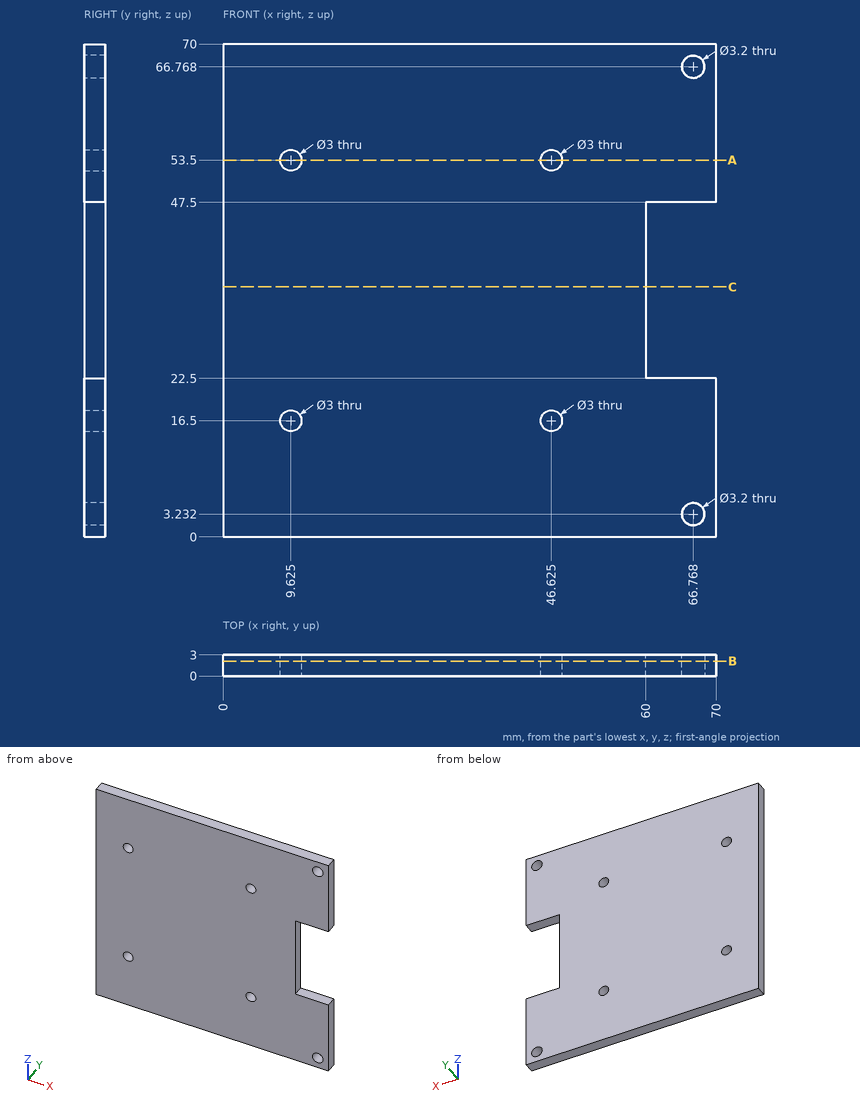
Study the drawing (mm; zero at the part's minimum x, y, z) and answer. Round coordinates to 2 decimals unless told otherwise and drop trailing zeros. Order: outer loops, then holes, each group sorted by start corner. A loop starts at its lowest first (then second) coordinate and runs counter-clockwise, first axis right, second up. Notation, with made-up numbers: (-40, -26) -> (-11, -26) arc R22 cw to (-11, -8) -> close; hole circle Ø11 at (89.25, 72). An arc over 180 degrees is marked (long way). Answer as CSV lines item,"result". Start each with the question number.
(1) The part is cut by section C-C (z = 35.5). Determine the outline of the cut face in (x, y).
(2) The part is cut by section B-B (y = 2.1). Determine the outline of the cut face in (x, z) (1 decimal).
(3) The part is cut by section A-A (z = 53.5). Determine the outline of the cut face in (x, y) (3 decimals), then the cut area to 3 significant figures.
(4) Find the intervals of material crossed by probe 1 along X at (y, z) = (0.7, 16.5) (3 decimals); probe 2 along X at (y, z) = (0.65, 3) (1 decimal); probe 3 along Z at (x, y) = (66, 2.2), in increasing order. Write a range as from..to.
Evaluation:
1,outline,"(0, 0) -> (60, 0) -> (60, 3) -> (0, 3) -> close"
2,outline,"(0, 0) -> (70, 0) -> (70, 22.5) -> (60, 22.5) -> (60, 47.5) -> (70, 47.5) -> (70, 70) -> (0, 70) -> close; hole circle Ø3 at (9.6, 16.5); hole circle Ø3 at (9.6, 53.5); hole circle Ø3 at (46.6, 16.5); hole circle Ø3 at (46.6, 53.5); hole circle Ø3.2 at (66.8, 3.2); hole circle Ø3.2 at (66.8, 66.8)"
3,outline,"(0, 0) -> (8.125, 0) -> (8.125, 3) -> (0, 3) -> close; (11.125, 0) -> (45.125, 0) -> (45.125, 3) -> (11.125, 3) -> close; (48.125, 0) -> (70, 0) -> (70, 3) -> (48.125, 3) -> close"
3,area,"192 mm²"
4,probe 1,"0..8.125, 11.125..45.125, 48.125..70"
4,probe 2,"0..65.2, 68.4..70"
4,probe 3,"0..1.83, 4.64..22.5, 47.5..65.36, 68.17..70"
